Could you check a few things on this model? Use its own coordinates, in mm. Give positions to 0.01 mm unless a question says otherwise; leave off trailing zeros. Write each loop counter-clockwise with the first axis right and the second up, starting at its lowest first coordinate (ties: lowest second). Pieces come first, ordered by that corner, then holes. Notation, with made-up numbers: (-39, 78) -> (6, 78) arc R29 ccw to (6, 113) -> close; hole circle Ø4 at (26.5, -23.5). An arc over 180 degrees is marked (long way). Write item = value, one per line. Start each with the question number.
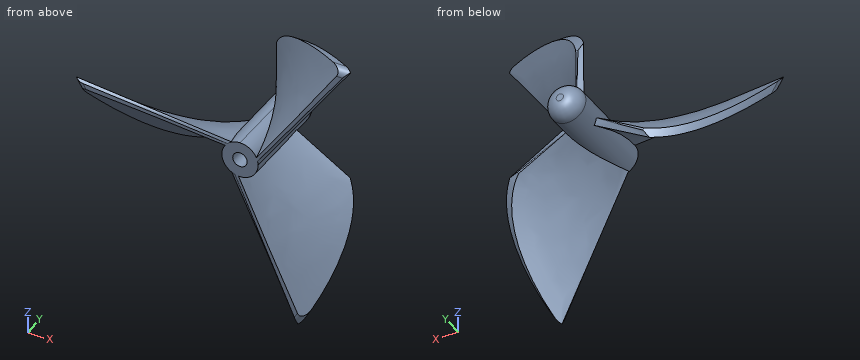
```python
from build123d import *

# Parameters (mm, degrees)
SKETCH1_R           = 2.5
BOSS_EXTRUDE1_DEPTH = 15
CUT_EXTRUDE1_START  = -4
CUT_EXTRUDE1_DEPTH  = 24
CIRPATTERN1_COUNT   = 3
SKETCH5_R           = 1
CUT_EXTRUDE2_DEPTH  = 8
FILLET1_R           = 2


with BuildPart() as part:
    # Sketch1 → Boss-Extrude1 (new body)
    with BuildSketch(Plane(origin=(0, 0, 0), x_dir=(1, 0, 0), z_dir=(0, 1, 0))):
        with Locations(Location((0, 0, 0), (0, 0, 270))):
            Circle(SKETCH1_R)
    extrude(amount=BOSS_EXTRUDE1_DEPTH)

    # Sketch2 → Loft1 section 0
    with BuildSketch(Plane.XY):
        with BuildLine():
            Line((-0.490290338, 9.901941932), (0.490290338, 10.098058068))
            Line((0.490290338, 10.098058068), (2.490290338, 0.098058068))
            Line((2.490290338, 0.098058068), (1.509709662, -0.098058068))
            Line((1.509709662, -0.098058068), (-0.490290338, 9.901941932))
        make_face()
    # Sketch3 → Loft1 section 1
    with BuildSketch(Plane.XY.offset(18)):
        with BuildLine():
            Line((0.277350098, 10.416025147), (-0.277350098, 9.583974853))
            Line((-0.277350098, 9.583974853), (14.722649902, -0.416025147))
            Line((14.722649902, -0.416025147), (15.277350098, 0.416025147))
            Line((15.277350098, 0.416025147), (0.277350098, 10.416025147))
        make_face()
    loft1 = loft()

    # Sketch4 → Cut-Extrude1 (cut)
    with BuildSketch(Plane(origin=(0, 0, 0), x_dir=(0, 0, -1), z_dir=(1, 0, 0)).offset(CUT_EXTRUDE1_START)):
        with BuildLine():
            Line((-2.5, 0), (-16.873666391, 0))
            ThreePointArc((-16.873666391, 0), (-17.638701098, 0.35601095), (-17.85901434, 1.170556207))
            ThreePointArc((-17.85901434, 1.170556207), (-15.190311544, 6.760544166), (-10, 10.141462099))
            Line((-10, 10.141462099), (-2.5, 10.141462099))
            Line((-2.5, 10.141462099), (-2.5, 10.760596561))
            Line((-2.5, 10.760596561), (-20.212640045, 10.760596561))
            Line((-20.212640045, 10.760596561), (-20.212640045, -1.946882985))
            Line((-20.212640045, -1.946882985), (-2.5, -1.111727068))
            Line((-2.5, -1.111727068), (0, -1.111727068))
            Line((0, -1.111727068), (0, 0))
            Line((0, 0), (-2.5, 0))
        make_face()
    cut_extrude1 = extrude(amount=CUT_EXTRUDE1_DEPTH, mode=Mode.SUBTRACT)

    # CirPattern1: Loft1, Cut-Extrude1 ×3 about axis
    cirpattern1_axis = Axis((0, 15, 0), (0, -1, 0))
    add([loft1.rotate(cirpattern1_axis, i * 360 / CIRPATTERN1_COUNT) for i in range(1, CIRPATTERN1_COUNT)])
    add([cut_extrude1.rotate(cirpattern1_axis, i * 360 / CIRPATTERN1_COUNT) for i in range(1, CIRPATTERN1_COUNT)], mode=Mode.SUBTRACT)

    # Sketch5 → Cut-Extrude2 (cut)
    with BuildSketch(Plane.XZ):
        with Locations(Location((0, 0, 0), (0, 0, 270))):
            Circle(SKETCH5_R)
    extrude(amount=-CUT_EXTRUDE2_DEPTH, mode=Mode.SUBTRACT)

    # Fillet1
    fillet1_edges = [part.edges().sort_by_distance(p)[0] for p in [
        (0, 15, -2.5),
    ]]
    fillet(fillet1_edges, radius=FILLET1_R)


solid = part.part
```
(1) Imagine slicing it at A-A (y = 11.25). Please give me the cut outline in (x, z).
(2) I'm going to push flat-ended pins straight in: pin 1 (4.5 mm diameter, centred on x = -4.5, z = -2.5, fed in from +Y); pin 2 (2 mm diameter, centred on x = 9.5, z = -10.5, fed in from +Y); pin 3 (5 mm diameter, centred on x = 3, y = 13.5, fed in from +Z). Where does each tip first touch, or does it pass through?
(3) If I drill on line 1 along X through (y, z) = (2, 13); line 2 along Y through (x, z) = (5.5, -16.5); line 3 along Z through (x, y) = (5.5, 9), over which ranges is the centre line in solid material (lowest first)? Write a range as from..to.
Answers below:
q1.outline = circle Ø5 at (0, 0)
q2.pin_1 = 10.14
q2.pin_2 = 7.78
q2.pin_3 = 2.44
q3.line_1 = 8.4..9.82
q3.line_2 = 0.14..0.5
q3.line_3 = -4.65..-3.3
